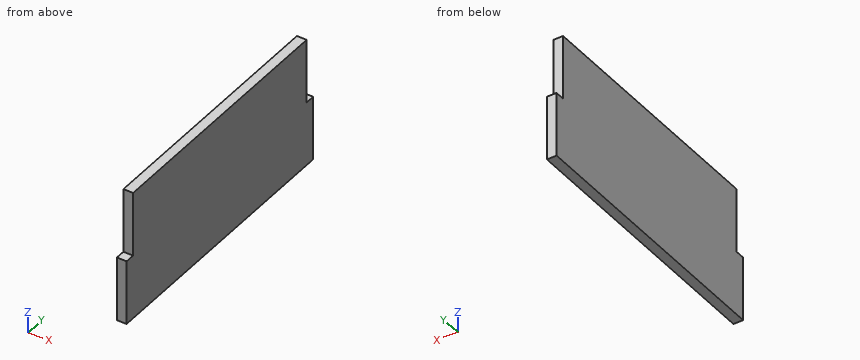
Solid Edge part; units mm, degrees
sketch "Sketch1" plane through (0, 0, 0) normal (1, 0, 0) x (0, 1, 0)
  line L0 (3, 40) -> (83, 40)
  line L1 (83, 40) -> (83, 20)
  line L2 (83, 20) -> (86, 20)
  line L3 (86, 20) -> (86, 0)
  line L4 (86, 0) -> (0, 0)
  line L5 (0, 0) -> (0, 20)
  line L6 (0, 20) -> (3, 20)
  line L7 (3, 20) -> (3, 40)
  dimension "D1" = 86
  dimension "D2" = 83
  dimension "D3" = 3
  dimension "D4" = 83
extrude "Protrusion1" add sketch "Sketch1" against normal blind 3
properties material "Acier"
Model file for the job. Use its own axes, mm. Coordinates: 2 decimals unless noted, no trailing zeros. Order: outer loops, then holes, each group sorted by start corner. A loop starts at its lowest first (then second) coordinate and runs counter-clockwise, first axis right, second up. Notation, with made-up numbers: (-17, 13.5) -> (15, 13.5) arc R26 ccw to (15, 45.5) -> close; hole circle Ø4 at (33.5, 79.25). An arc over 180 degrees is marked (long way). Answer as a JSON object with one key per item and string values. Group by question number.
1) Cut at B-B, the plane z = 34. Write the cut outline in (x, y), then the cut area to 3 significant figures.
2) Flat gauge pins, fed straight in: pin 1 (4 mm diameter, centred on y = 49, z = 13.5, fed in from +X); pin 2 (1.5 mm diameter, centred on x = -1.5, z = 34, fed in from +Y); pin 3 (0.9 mm diameter, centred on x = -1, y = 1, fed in from +Z); pin 4 (1.5 mm diameter, centred on x = -1, z = 31, fed in from -Y). Where does each tip first touch, or does it go through?
3) Drill centre line: L1, parallel to Y at x = -2.15, z = 22.5. Where is it in solid material? Low to high.
4) Cut at A-A, the plane x = -1.15. Write the cut outline in (y, z).
Check values:
{
 "1": {"outline": "(-3, 3) -> (0, 3) -> (0, 83) -> (-3, 83) -> close", "area": "240 mm²"},
 "2": {"pin 1": "stops at x = 0", "pin 2": "stops at y = 83", "pin 3": "stops at z = 20", "pin 4": "stops at y = 3"},
 "3": {"L1": "y = 3 to 83"},
 "4": {"outline": "(0, 0) -> (86, 0) -> (86, 20) -> (83, 20) -> (83, 40) -> (3, 40) -> (3, 20) -> (0, 20) -> close"}
}
